```python
from build123d import *

# Parameters (mm, degrees)
F0_W     = 34
F0_H     = 40
F1_DEPTH = 40
F2_W     = 27
F2_H     = 35
F3_DEPTH = 35
F5_DEPTH = 34.001
F7_DEPTH = 5.001
F9_DEPTH = 5.001
F10_R    = 1.5


with BuildPart() as f1:
    # F0 (on Top) → F1 (new body)
    with BuildSketch(Plane.XY):
        Rectangle(F0_W, F0_H)
    extrude(amount=F1_DEPTH)

    # F2 (on face) → F3 (cut)
    with BuildSketch(Plane.XZ.offset(20)):
        with Locations((0, 22.5)):
            Rectangle(F2_W, F2_H)
    extrude(amount=-F3_DEPTH, mode=Mode.SUBTRACT)

    # F4 (on face) → F5 (cut, through all)
    with BuildSketch(Plane(origin=(-17, 0, 0), x_dir=(0, -1, 0), z_dir=(-1, 0, 0))):
        Polygon((20, 40), (-12, 40), (-12, 35), (15, 8), (20, 8), align=None)
    extrude(amount=-F5_DEPTH, mode=Mode.SUBTRACT)

    # F6 (on face) → F7 (cut, through all)
    with BuildSketch(Plane.XY.offset(5)):
        with BuildLine():
            ThreePointArc((4.25, 8), (0, 3.75), (-4.25, 8))
            Line((-4.25, 8), (-4.25, -8))
            ThreePointArc((-4.25, -8), (0, -3.75), (4.25, -8))
            Line((4.25, -8), (4.25, 8))
        make_face()
        with BuildLine():
            ThreePointArc((4.25, 8), (3.00520382, 11.00520382), (0, 12.25))
            ThreePointArc((0, 12.25), (-3.00520382, 11.00520382), (-4.25, 8))
            ThreePointArc((-4.25, 8), (0, 3.75), (4.25, 8))
        make_face()
        with BuildLine():
            ThreePointArc((4.25, -8), (0, -3.75), (-4.25, -8))
            ThreePointArc((-4.25, -8), (-3.00520382, -11.00520382), (0, -12.25))
            ThreePointArc((0, -12.25), (3.00520382, -11.00520382), (4.25, -8))
        make_face()
    extrude(amount=-F7_DEPTH, mode=Mode.SUBTRACT)

    # F8 (on face) → F9 (cut, through all)
    with BuildSketch(Plane.XZ.offset(-15)):
        with BuildLine():
            ThreePointArc((4.25, 28), (0, 23.75), (-4.25, 28))
            Line((-4.25, 28), (-4.25, 12))
            ThreePointArc((-4.25, 12), (0, 16.25), (4.25, 12))
            Line((4.25, 12), (4.25, 28))
        make_face()
        with BuildLine():
            ThreePointArc((4.25, 28), (3.00520382, 31.00520382), (0, 32.25))
            ThreePointArc((0, 32.25), (-3.00520382, 31.00520382), (-4.25, 28))
            ThreePointArc((-4.25, 28), (0, 23.75), (4.25, 28))
        make_face()
        with BuildLine():
            ThreePointArc((4.25, 12), (0, 16.25), (-4.25, 12))
            ThreePointArc((-4.25, 12), (-3.00520382, 8.99479618), (0, 7.75))
            ThreePointArc((0, 7.75), (3.00520382, 8.99479618), (4.25, 12))
        make_face()
    extrude(amount=-F9_DEPTH, mode=Mode.SUBTRACT)

    # F10
    f10_edges = [f1.edges().sort_by_distance(p)[0] for p in [
        (-15.25, -15, 8),
        (15.25, -15, 8),
        (15.25, -20, 8),
        (-15.25, -20, 8),
        (15.25, 12, 35),
        (-15.25, 12, 35),
        (-15.25, 12, 40),
        (15.25, 12, 40),
    ]]
    fillet(f10_edges, radius=F10_R)


solid = f1.part
```
Build history of the part. All positions in model axes, mm. A direction names the side the tool comes from. Round coordinates to 2 decimals unless told otherwise and drop trailing zeros. Order: outer loops, then holes, each group sorted by start corner. A loop starts at its lowest first (then second) coordinate and runs counter-clockwise, first axis right, second up. Notation, with made-up numbers: (-31.5, 36.5) -> (12.5, 36.5) arc R22 cw to (12.5, 70.5) -> close; hole circle Ø9 at (55.25, 65.5). An arc over 180 degrees is marked (long way). Answer in a Markdown table with one row per item.
1) Band-saw the part on A-A on y = 6.5. Give the cut face in (x, z), and give its area (3 significant figures).
Values:
| item | result |
|---|---|
| outline | (-17, 0) -> (-4.25, 0) -> (-4.25, 5) -> (-13.5, 5) -> (-13.5, 29.5) -> (-17, 29.5) -> close; (4.25, 0) -> (17, 0) -> (17, 29.5) -> (13.5, 29.5) -> (13.5, 5) -> (4.25, 5) -> close |
| area | 299 mm2 |
2) Mould opens along X. For faces 1 (the flat face through (4.25, 17, 20)), 2 (the flat face through (-13.5, 5, 14)), 3 (the cylindrical face through (15.27, -19.57, 7.55)), 4 (the flat face through (17, 4, 15)) say: released by +X, released by -X, zero draft, split by the parting line, or undercut.
Values:
| item | result |
|---|---|
| face 1 | undercut |
| face 2 | undercut |
| face 3 | zero draft |
| face 4 | released by +X |
3) Band-saw the part on B-B on z = 14. Give the cut face in (x, y).
Values:
| item | result |
|---|---|
| outline | (-17, -9) -> (-13.5, -9) -> (-13.5, 15) -> (-4.25, 15) -> (-4.25, 20) -> (-17, 20) -> close; (4.25, 15) -> (13.5, 15) -> (13.5, -9) -> (17, -9) -> (17, 20) -> (4.25, 20) -> close |
4) Pin check, flat tips, straight feed: P1, Ø6, axis at x = 2, y = 9.5, coming from the -Z side; P2, Ø13.5, axis at x = 1, y = -1.5, coming from the +Z side; P3, Ø4, axis at x = 7, z = 18.5, coming from the -Y side; P4, Ø0.9, axis at x = -14.5, y = -17.5, coming from the +Z side. Stop position of each tip, or through.
Values:
| item | result |
|---|---|
| P1 | z = 0 |
| P2 | z = 5 |
| P3 | y = 15 |
| P4 | z = 8 |
5) Band-saw the part on C-C on x = 8. Give the cut face in (y, z).
Values:
| item | result |
|---|---|
| outline | (-20, 0) -> (20, 0) -> (20, 40) -> (15, 40) -> (15, 5) -> (-20, 5) -> close |
6) Band-saw the part on D-D on z = 34. Give the cut face in (x, y).
Values:
| item | result |
|---|---|
| outline | (-17, 11) -> (-13.5, 11) -> (-13.5, 15) -> (13.5, 15) -> (13.5, 11) -> (17, 11) -> (17, 20) -> (-17, 20) -> close |
7) Which spindle directions (+Z, -Z, +X, -X, +Y, -Y) get a long thin tool onto all of the face, cutting with end or side? Do faces 5 (the flat face through (7, 0, 0)), 6 (the flat face through (-4.25, 17, 20)), 7 (the flat face through (-4.25, 0, 3)), 8 (the flat face through (6, -3, 5)), 9 (the flat face through (-15, -17, 8)). Say none if no direction does.
Values:
| item | result |
|---|---|
| face 5 | -Z, +X, -X, +Y, -Y |
| face 6 | +Y, -Y |
| face 7 | +Z, -Z |
| face 8 | +Z, -Y |
| face 9 | +Z, +X, -X, -Y |
8) Wall check: L1, parallel to X at y = 0, z = 17; L2, parallel to X at y = 15.5, z = 27.5; L3, parallel to Z at x = 1, y = 14. Give the ranges that are in metal, low to high.
Values:
| item | result |
|---|---|
| L1 | -17 to -13.5, 13.5 to 17 |
| L2 | -17 to -4.25, 4.25 to 17 |
| L3 | 0 to 5 |
